Work out the finished part from the listing and answer in its coordinate system (mm). Coordinates: 2 decimals unless noted, no trailing zeros. Write each loop counter-clockwise with the first axis right and the second up, starting at its lowest first coordinate (ties: lowest second). Pieces come first, ordered by that corner, then holes. Notation, with made-up numbers: (34.5, 2.25) - (67.5, 2.25) arc R21 cw to (67.5, 17.25) - close; hole circle Ø1 at (65, 19.25). An arc over 180 degrees is marked (long way). Use one line per item in the form item = value. Start each with the question number.
Item 1: Consider probe 1 along Z at (x, y) = (26, 1.55); probe 2 along Z at (x, y) = (-26, 2.25); probe 3 along X at (y, z) = (1.15, -21.5). Determine where each line is inside the solid, lowest interval first.
Item 2: Determine the mould class of faces 1 (the flat face through (-7, 3, -19)), 2 (the cylindrical face through (-28.48, 0.45, -24.43)), 3 (the cylindrical face through (-6.66, 1.48, -0.06)) for opening direction Y: released by +Y, released by -Y, zero draft, split by the parting line, or undercut.
Item 3: Given pin 1 (1 mm diameter, centred on y = 2, z = -44, fed in from +X), flat-ended and moving along its own axis, determine where the tip first touches the part or whether it passes through.
Item 4: A cutting plane is placed at A-A (y = 0.5). Write down the section's boundary in (x, z).
from build123d import *

# Parameters (mm, degrees)
EXTRUDE_1_DEPTH          = 3
FILLET_1_R               = 1.5
CUT_EXTRUDE_1_DEPTH      = 69.078755293
CUT_EXTRUDE_1_DEPTH_BACK = 69.078755293
SKETCH_2_R               = 19


with BuildPart() as part:
    # Эскиз1 → Бобышка-Вытянуть1 (new body)
    with BuildSketch(Plane(origin=(0, 0, 0), x_dir=(1, 0, 0), z_dir=(0, 1, 0))):
        Polygon((-46.105497744, 0), (33.894502256, 0), (-1.105497744, 50), (-11.105497744, 50), align=None)
    extrude(amount=EXTRUDE_1_DEPTH)

    # Скругление1
    fillet_1_edges = [part.edges().sort_by_distance(p)[0] for p in [
        (16.394502256, 0, -25),
        (16.394502256, 3, -25),
        (-28.605497744, 0, -25),
        (-28.605497744, 3, -25),
        (-6.105497744, 0, -50),
        (-6.105497744, 3, -50),
    ]]
    fillet(fillet_1_edges, radius=FILLET_1_R - 0.0001)  # a hair under: the kernel refuses the full size

    # Эскиз2 → Вырез-Вытянуть1 (cut, two sides: drawn at the far end of the back side and taken through both)
    with BuildSketch(Plane(origin=(0, 0, 0), x_dir=(0, 0, -1), z_dir=(1, 0, 0)).offset(-CUT_EXTRUDE_1_DEPTH_BACK)):
        with Locations((-18.940696925, 1.5)):
            Circle(SKETCH_2_R)
    extrude(amount=CUT_EXTRUDE_1_DEPTH + CUT_EXTRUDE_1_DEPTH_BACK, mode=Mode.SUBTRACT)


solid = part.part
Answer:
q1.probe_1 = -11.28 to -0.06
q1.probe_2 = -28.37 to -0.04
q1.probe_3 = -31 to 18.79
q2.face_1 = released by +Y
q2.face_2 = released by -Y
q2.face_3 = undercut
q3.pin_1 = 3.38
q4.outline = (-45.62, -0.03) - (-10.91, -49.62) - (-1.3, -49.62) - (33.41, -0.03) - close
